```python
from build123d import *

# Parameters (mm, degrees)
SKETCH1_W           = 26.2
SKETCH1_H           = 46.8
SKETCH1_W_2         = 20.2
SKETCH1_H_2         = 40.8
BOSS_EXTRUDE1_DEPTH = 25
SKETCH3_W           = 10.2
SKETCH3_H           = 25
CUT_EXTRUDE1_DEPTH  = 10
FILLET1_R           = 0.5
SKETCH4_W           = 26.2
SKETCH4_H           = 46.8
BOSS_EXTRUDE2_DEPTH = 2
FILLET2_R           = 1


with BuildPart() as part:
    # Sketch1 → Boss-Extrude1 (new body)
    with BuildSketch(Plane(origin=(0, 0, 0), x_dir=(1, 0, 0), z_dir=(0, 1, 0))):
        with Locations((13.1, 23.4)):
            Rectangle(SKETCH1_W, SKETCH1_H)
        with Locations((13.1, 23.4)):
            Rectangle(SKETCH1_W_2, SKETCH1_H_2, mode=Mode.SUBTRACT)
    extrude(amount=BOSS_EXTRUDE1_DEPTH)

    # Sketch3 → Cut-Extrude1 (cut)
    with BuildSketch(Plane.XY):
        with Locations((13.1, 12.5)):
            Rectangle(SKETCH3_W, SKETCH3_H)
    extrude(amount=-CUT_EXTRUDE1_DEPTH, mode=Mode.SUBTRACT)

    # Fillet1
    fillet1_edges = [part.edges().sort_by_distance(p)[0] for p in [
        (3, 0, -23.4),
        (5.5, 0, -3),
        (23.2, 0, -23.4),
        (13.1, 0, -43.8),
        (3, 25, -23.4),
        (5.5, 25, -3),
        (23.2, 25, -23.4),
        (13.1, 25, -43.8),
        (20.7, 0, -3),
        (20.7, 25, -3),
    ]]
    fillet(fillet1_edges, radius=FILLET1_R)

    # Sketch4 → Boss-Extrude2 (add)
    with BuildSketch(Plane(origin=(0, 25, 0), x_dir=(1, 0, 0), z_dir=(0, 1, 0))):
        with Locations((13.1, 23.4)):
            Rectangle(SKETCH4_W, SKETCH4_H)
    extrude(amount=BOSS_EXTRUDE2_DEPTH)

    # Fillet2
    fillet2_edges = [part.edges().sort_by_distance(p)[0] for p in [
        (0, 13.5, -46.8),
        (26.2, 13.5, -46.8),
        (26.2, 13.5, 0),
        (0, 13.5, 0),
    ]]
    fillet(fillet2_edges, radius=FILLET2_R)


solid = part.part
```
Source: CAD feature listing. Evaluate the final solid. Frame: model axes, mm. A direction names the side the tool comes from. Coordinates: 2 decimals unless noted, no trailing zeros. Write each loop counter-clockwise with the first axis right and the second up, starting at its lowest first coordinate (ties: lowest second). Pieces come first, ordered by that corner, then holes. Notation, with made-up numbers: (43, -1.75) -> (94, -1.75) arc R14 ccw to (94, 18.25) -> close; hole circle Ø1 at (-1.5, 24). An arc over 180 degrees is marked (long way). Return JSON: item names as keys, results as strings. Group by question number.
1) Section query A-A, the plane z = -5. Return loops of the section in (x, y).
2) Ray query, line 1 along X through (y, z) = (24, -19.5); line 2 along Z through (x, y) = (4.5, 14); line 3 along Z through (x, y) = (17, 16.5). Return the intervals inside material, ascending.
3) Section query C-C, the plane x = 17.25. Return loops of the section in (y, z), plus the area to 3 significant figures.
4) Set-up query: faces 4 (the face through (18.2, 12, -1)), 5 (the face through (23.2, 12, -23)), 6 (the face through (0.285, 13.311, -46.499)). Return all of +Z, -Z, +X, -X, +Y, -Y with unobstructed straight access to the full face (end or side cutting, diameter ignored); none if empty.
5) Contact query for a flat-ended pin moving along its axis: P1, Ø1, axis at x = 19.5, z = -11.5, coming from the -Y side. Output: stop coordinate, or through.
6) Mould query, pull axis X, two halves, no side actions, for faces 1 (the face through (5, 12, -3)), 2 (the face through (0.285, 13.689, -0.301)), 3 (the face through (25.915, 13.311, -46.499)). Classes: +X half, -X half, draft (parallel to the pull), parting line (faces both ways), or undercut.
7) Section query D-D, the plane x = 3.5. Return loops of the section in (y, z).
8) Section query B-B, the plane y = 7.5. Return loops of the section in (x, z).
From the geometry:
{
 "1": {"outline": "(0, 0) -> (2.5, 0) arc R0.5 ccw to (3, 0.5) -> (3, 24.5) arc R0.5 ccw to (2.5, 25) -> (23.7, 25) arc R0.5 ccw to (23.2, 24.5) -> (23.2, 0.5) arc R0.5 ccw to (23.7, 0) -> (26.2, 0) -> (26.2, 27) -> (0, 27) -> close"},
 "2": {"line 1": "0 to 3, 23.2 to 26.2", "line 2": "-46.8 to -43.8, -3 to 0", "line 3": "-46.8 to -43.8"},
 "3": {"outline": "(0, -46.8) -> (27, -46.8) -> (27, 0) -> (25, 0) -> (25, -44.3) arc R0.5 ccw to (24.5, -43.8) -> (0.5, -43.8) arc R0.5 ccw to (0, -44.3) -> close", "area": "168 mm²"},
 "4": {"face 4": "+Z, -Y", "face 5": "-Y", "face 6": "-Z, -X, +Y, -Y"},
 "5": {"P1": "y = 25"},
 "6": {"face 1": "undercut", "face 2": "-X half", "face 3": "+X half"},
 "7": {"outline": "(0, -46.8) -> (27, -46.8) -> (27, 0) -> (0, 0) -> (0, -2.5) arc R0.5 ccw to (0.5, -3) -> (24.5, -3) arc R0.5 ccw to (25, -2.5) -> (25, -44.3) arc R0.5 ccw to (24.5, -43.8) -> (0.5, -43.8) arc R0.5 ccw to (0, -44.3) -> close"},
 "8": {"outline": "(0, -45.8) arc R1 ccw to (1, -46.8) -> (25.2, -46.8) arc R1 ccw to (26.2, -45.8) -> (26.2, -1) arc R1 ccw to (25.2, 0) -> (18.2, 0) -> (18.2, -3) -> (23.2, -3) -> (23.2, -43.8) -> (3, -43.8) -> (3, -3) -> (8, -3) -> (8, 0) -> (1, 0) arc R1 ccw to (0, -1) -> close"}
}
